Can you work these out from the model? Positions are in its coordinate system, mm. Give positions to 0.01 mm unless a question says otherwise; leave off trailing zeros. Order: outer loops, then holes, each group sorted by start corner. A loop starts at its lowest first (then second) coordinate and runs counter-clockwise, first axis right, second up. Notation, with made-up numbers: (78, -16) - (84, -16) arc R21 cw to (84, 17) - close; hole circle Ø5 at (42.25, -12). An arc over 180 degrees is marked (long way). Return JSON: item names as keys, results as strings.
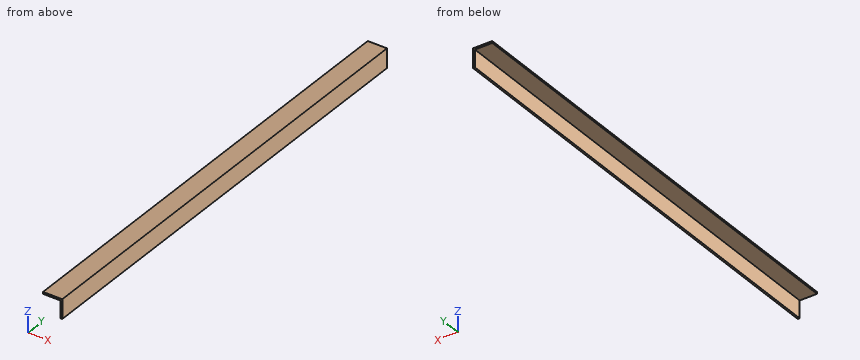
Autodesk Inventor part; units mm, degrees
ref_plane "YZ Plane" through (0, 0, 0) normal (1, 0, 0) x (0, 1, 0)
ref_plane "XZ Plane" through (0, 0, 0) normal (0, 1, 0) x (-1, 0, 0)
ref_plane "XY Plane" through (0, 0, 0) normal (0, 0, 1) x (1, 0, 0)
sketch "Sketch1" plane through (0, 0, 0) normal (0, 1, 0) x (-1, 0, 0)
  line L0 (38.8889, 27.7778) -> (-11.1111, 27.7778)
  line L1 (-11.1111, 27.7778) -> (-11.1111, -22.2222)
  line L2 (38.8889, 27.7778) -> (38.8889, 22.7778)
  line L3 (38.8889, 22.7778) -> (-6.1111, 22.7778)
  line L4 (-6.1111, 22.7778) -> (-6.1111, -22.2222)
  line L5 (-6.1111, -22.2222) -> (-11.1111, -22.2222)
  point P0 (0, 0)
  dimension "d0" = 50
  dimension "d1" = 50
  dimension "d2" = 5
  dimension "d3" = 5
extrude "Extrusion1" add sketch "Sketch1" along normal blind 1200
properties part number "Ugol800"
1. For pin 1 Ø12 at (y, z) = (250.5, -15.5) entering from -X; pin 2 Ø1.5 at (x, z) = (4, 19) entering from -Y, each with a flat end and sliding along its axis, tell me the tip position at first contact or that it passes through.
Checks:
{"pin 1": "x = 6.11", "pin 2": "through"}
2. Suppose I cut it at B-B (z = 11.5). List the corners of the cut face in (x, y) for me, plus the area to 3 significant figures.
Checks:
{"outline": "(6.11, 0) - (11.11, 0) - (11.11, 1200) - (6.11, 1200) - close", "area": "6,000 mm^2"}
3. If I drill on L1, parallel to X at y = 315, z = -5; L2, parallel to Z at x = -10.5, y = 440, over which ranges is the centre line in solid material (lowest first)? Write a range as [from, to].
Checks:
{"L1": "[6.11, 11.11]", "L2": "[22.78, 27.78]"}
4. Suppose I cut it at C-C (x = -21.5). List the corners of the cut face in (y, z) for me, plus the area to 3 significant figures.
Checks:
{"outline": "(0, 22.78) - (1200, 22.78) - (1200, 27.78) - (0, 27.78) - close", "area": "6,000 mm^2"}
5. Suppose I cut it at A-A (y = 640). List the corners of the cut face in (x, z) for me, plus the area to 3 significant figures.
Checks:
{"outline": "(-38.89, 22.78) - (6.11, 22.78) - (6.11, -22.22) - (11.11, -22.22) - (11.11, 27.78) - (-38.89, 27.78) - close", "area": "475 mm^2"}
